Autodesk Inventor part; units mm, degrees
ref_plane "YZ Plane" through (0, 0, 0) normal (1, 0, 0) x (0, 1, 0)
ref_plane "XZ Plane" through (0, 0, 0) normal (0, 1, 0) x (-1, 0, 0)
ref_plane "XY Plane" through (0, 0, 0) normal (0, 0, 1) x (1, 0, 0)
sketch "Sketch1" plane through (0, 0, 0) normal (0, 1, 0) x (-1, 0, 0)
  circle A0 centre (0, 0) radius 1.925
  dimension "d0" = 3.85
extrude "Extrusion1" add sketch "Sketch1" along normal blind 2.5
sketch "Sketch2" plane through (0, 2.5, 0) normal (0, 1, 0) x (1, 0, 0)
  line L0 (-1, -3) -> (1, -3)
  line L1 (3, -1) -> (3, 1)
  line L2 (1, 3) -> (-1, 3)
  line L3 (-3, 1) -> (-3, -1)
  line L4 (-3, -3) -> (3, 3) construction
  line L5 (3, -3) -> (-3, 3) construction
  arc A0 (-3, -1) -> (-1, -3) centre (-1, -1) ccw
  arc A1 (-1, 3) -> (-3, 1) centre (-1, 1) ccw
  arc A2 (3, 1) -> (1, 3) centre (1, 1) ccw
  arc A3 (1, -3) -> (3, -1) centre (1, -1) ccw
  point P0 (0, 0)
  dimension "d3" = 6
  dimension "d4" = 6
  dimension "d5" = 2
extrude "Extrusion2" add sketch "Sketch2" along normal blind 2
sketch "Sketch3" plane through (0, 4.5, 0) normal (0, 1, 0) x (1, 0, 0)
  circle A0 centre (0, 0) radius 1.925
extrude "Extrusion3" add sketch "Sketch3" along normal blind 2
sketch "Sketch5" plane through (0, 6.5, 0) normal (0, 1, 0) x (1, 0, 0)
  circle A0 centre (0, 0) radius 3.5
  dimension "d14" = 7
extrude "Extrusion5" add sketch "Sketch5" along normal blind 2
sketch "Sketch6" plane through (0, 8.5, 0) normal (0, 1, 0) x (1, 0, 0)
  circle A0 centre (0, 0) radius 1.925
extrude "Extrusion6" add sketch "Sketch6" along normal blind 5
sketch "Sketch7" plane through (0, 13.5, 0) normal (0, 1, 0) x (1, 0, 0)
  circle A0 centre (0, 0) radius 3.5
extrude "Extrusion7" add sketch "Sketch7" along normal blind 2
sketch "Sketch8" plane through (0, 4.5, 0) normal (0, 1, 0) x (1, 0, 0)
  circle A0 centre (0, 0) radius 1.925
  arc A1 (1, -3) -> (3, -1) centre (1, -1) ccw
  line L0 (3, -1) -> (3, 1)
  arc A2 (3, 1) -> (1, 3) centre (1, 1) ccw
  line L1 (1, 3) -> (-1, 3)
  arc A3 (-1, 3) -> (-3, 1) centre (-1, 1) ccw
  line L2 (-3, 1) -> (-3, -1)
  arc A4 (-3, -1) -> (-1, -3) centre (-1, -1) ccw
  line L3 (-1, -3) -> (1, -3)
loft "Loft1" add section 1 edges at (2.4142, 4.5, 2.4142) (3, 4.5, 0) (2.4142, 4.5, -2.4142) (0, 4.5, -3) (-2.4142, 4.5, -2.4142) (-3, 4.5, 0) (-2.4142, 4.5, 2.4142) (0, 4.5, 3) section 2 edges at (-3.5, 6.5, 0)
fillet "Fillet3" radius 1 5 edges at (-3.5, 8.5, 0) (-1.925, 8.5, 0) (-1.925, 13.5, 0) (-3.5, 13.5, 0) (-3.5, 15.5, 0)
properties part number "guia"
Geometry: final body of the model. Coordinates: model frame, mm. A direction names the side the tool comes from. Give positions to 0.01 mm unless a question says otherwise; leave off trailing zeros. Loops run counter-clockwise (first coordinate to the right, second up) from the corner with the lowest first, then second, coordinate; pieces in that order, holes last. Notation, with made-up numbers: M 63.25,24 L 94.25,24 A25 cw 94.25,63 Z; hole C 12.5,24 d7. An arc over 180 degrees is marked long. Put each result on its own line as item: value.
1) First-contact query: P1, Ø1, axis at x = 0, y = 3, coming from the +Z side; P2, Ø1, axis at y = 8, z = 2, coming from the -X side; P3, Ø3, axis at y = 5.5, z = -2.5, coming from the +X side. Flat tips, straight axial feed; report the tip coordinate or a pass-through.
Computed values:
P1: stops at z = 3
P2: stops at x = -3.09
P3: stops at x = 3.25
2) Reachability of faces 1 (the flat face through (-3, 3, 0)), 2 (the cylindrical face through (-2.43, 3.49, -2.4)), 3 (the cylindrical face through (2.43, 3.49, 2.4)), 4 (the cylindrical face through (0.42, 1.23, 1.88)) from +Z, -Z, +X, -X, +Y, -Y: full face, straight path, thin tool, end or side. Return the list, or none.
Computed values:
face 1: +Z, -Z, -X, -Y
face 2: -Z, -X, -Y
face 3: +Z, +X, -Y
face 4: -Y
3) Material intervals for L1, parallel to Y at x = 2.5, z = -0.75; L2, parallel to X at y = 10.25, z = 0 (3 decimals); L3, parallel to Y at x = -1, z = 1.75, sorted ascending. Write a range as from..to.
Computed values:
L1: y = 2.5..8.51, 13.45..15.49
L2: x = -1.925..1.925
L3: y = 2.5..9.04, 12.92..15.5
4) Cut plane A-A, the plane y = 13. Return the cut outline in (x, z).
Computed values:
outline: C 0,0 d4.12
